from build123d import *

# Parameters (mm, degrees)
SKETCH2_OUTSIDE_W  = 20.924
SKETCH2_OUTSIDE_H  = 20.924
CUT_EXTRUDE1_DEPTH = 6.4
CHAMFER1_SIZE      = 0.5


with BuildPart() as part:
    # Sketch1 → Revolve1 (revolve)
    with BuildSketch(Plane(origin=(0, 0, 0), x_dir=(0, 0, -1), z_dir=(1, 0, 0)), mode=Mode.PRIVATE) as revolve1_sk:
        Polygon((3.2, 3.2), (3.2, -3.2), (6.25, -3.2), (7.3, -2.593782217), (7.3, 2.593782217), (6.25, 3.2), align=None)
    revolve(revolve1_sk.sketch.rotate(Axis((0, 12.02962963, 0), (0, -1, 0)), 180), axis=Axis((0, 12.02962963, 0), (0, -1, 0)))

    # Sketch2 outside → Cut-Extrude1 (cut)
    with BuildSketch(Plane(origin=(0, 3.2, 0), x_dir=(1, 0, 0), z_dir=(0, 1, 0))):
        Rectangle(SKETCH2_OUTSIDE_W, SKETCH2_OUTSIDE_H)
        Polygon((7.332348419, 0), (3.666174209, 6.35), (-3.666174209, 6.35), (-7.332348419, 0), (-3.666174209, -6.35), (3.666174209, -6.35), align=None, mode=Mode.SUBTRACT)
    extrude(amount=-CUT_EXTRUDE1_DEPTH, mode=Mode.SUBTRACT)

    # Chamfer1
    chamfer1_edges = [part.edges().sort_by_distance(p)[0] for p in [
        (0, -3.2, -3.2),
        (0, 3.2, -3.2),
    ]]
    chamfer(chamfer1_edges, length=CHAMFER1_SIZE)


solid = part.part
Design review of the part built by this model. Coordinates are the model's own, in mm. Give positions to 0.01 mm unless a question says otherwise; leave off trailing zeros. Loops run counter-clockwise (first coordinate to the right, second up) from the corner with the lowest first, then second, coordinate; pieces in that order, holes last. Notation, with made-up numbers: (77, -7) -> (115, -7) arc R11 ccw to (115, -2) -> close; hole circle Ø8 at (-30.5, -9). An arc over 180 degrees is marked (long way). One line per question, with ' | ' between items. Start each with the question number.
(1) Insertion check: P1, Ø1.5, axis at x = -4.5, y = -1.5, coming from the -Z side; P2, Ø5, axis at x = -0.5, z = 2, coming from the -Y side; P3, Ø1, axis at x = -4.5, y = 0, coming from the +Z side. Each pin has a flat end and moves straight along its axis. Give the tip position at first contact, or say it passes through.
(2) We need section A-A (x = 0). State the section outline as (y, z) points.
(3) For line 1 (X direction, y = 1.6, z = 0); line 2 (X direction, y = 1.25, z = 2.75); line 3 (Z direction, x = 1, y = -0.25), list the stretches that pass through material, from the lowest coordinate up.
(4) Draft analysis for pull direction X (two halves, no side actions). For faces 1 (the face through (0, 0, -6.35)), 2 (the face through (-5.524, 0.044, 3.131)), 3 (the face through (-0.961, -0.038, 3.052)), state which applies: +X half, -X half, draft (parallel to the pull), parting line (faces both ways), or undercut.
(5) We need section B-B (y = -2). State the section outline as (x, z) points, and give its area (3 significant figures).
The answers:
1) P1: stops at z = -6.2 | P2: stops at y = -3.2 | P3: stops at z = 5.77
2) outline: (-3.2, -6.25) -> (-3.14, -6.35) -> (3.14, -6.35) -> (3.2, -6.25) -> (3.2, -3.7) -> (2.7, -3.2) -> (-2.7, -3.2) -> (-3.2, -3.7) -> close; (-3.2, 3.7) -> (-2.7, 3.2) -> (2.7, 3.2) -> (3.2, 3.7) -> (3.2, 6.25) -> (3.14, 6.35) -> (-3.14, 6.35) -> (-3.2, 6.25) -> close
3) line 1: x = -7.3 to -3.2, 3.2 to 7.3 | line 2: x = -5.74 to -1.64, 1.64 to 5.74 | line 3: z = -6.35 to -3.04, 3.04 to 6.35
4) face 1: draft | face 2: -X half | face 3: undercut
5) outline: (-7.3, -0.06) -> (-3.7, -6.29) arc R7.3 ccw to (-3.6, -6.35) -> (3.6, -6.35) arc R7.3 ccw to (3.7, -6.29) -> (7.3, -0.06) arc R7.3 ccw to (7.3, 0.06) -> (3.7, 6.29) arc R7.3 ccw to (3.6, 6.35) -> (-3.6, 6.35) arc R7.3 ccw to (-3.7, 6.29) -> (-7.3, 0.06) arc R7.3 ccw to start; hole circle Ø6.4 at (0, 0) | area: 108 mm^2
